Study the drawing (mm; zero at the part's minimum x, y, z) and answer. A direction names the side the tool comes from. Coordinates: 2 decimals unless noted, no trailing zeros. Write each loop counter-clockwise with the first axis right and the second up, starting at its lowest first coordinate (ties: lowest second). Pieces come first, ordered by that corner, then holes. Notation, with made-up numbers: M 77.25,78.5 L 120.25,78.5 A20 cw 120.25,112.5 Z; hole C 79,41 d3. An arc over 180 degrees is marked long. Answer as a JSON object with one key per item and string values. Group by question number.
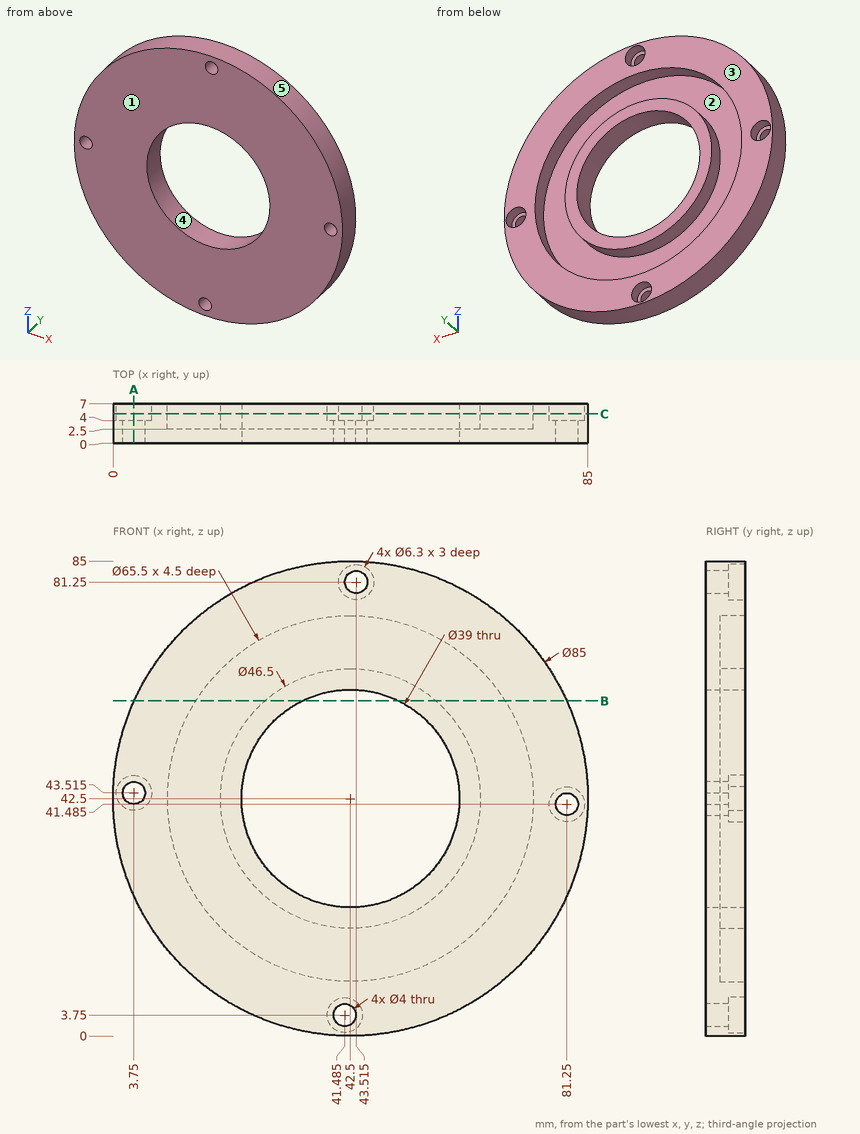
Item 1: A tool of negligible diameter and unlimited length cuts with its end or side. For the marked faces 1 and 2, from which of +Z, -Z, +X, -X, +Y, -Y can it reach the whole face along a straight path? Write none if from no direction.
Item 2: A cutting plane is placed at C-C, the plane y = 5.25. State how many separate pieces and enclosed holes the cut face has, and give its area (3 significant figures).
Item 3: Flat-ended cylindrical pins translate along their axes: pin 1 Ø3 at (x, y) = (29.5, 4.5) entering from +Z (1 decimal); pin 2 Ø1.9 at (x, z) = (42, 81.5) entering from +Y; pin 3 Ø3 at (x, y) = (16, 3) entering from +Z. Find the tip coordinate at first contact, or state that the pin passes through.
Item 4: A cutting plane is placed at B-B, the plane z = 60. Write down the section's boundary in (x, y).
Item 5: For a pull along Z with two mould halves and no side action, classify the marked faces 3, 4 and 5 as +Z half, -Z half, draft (parallel to the pull), parting line (faces both ways), or undercut.
Item 6: A cutting plane is placed at A-A, the plane x = 3.75. Write down the section's boundary in (y, z) (1 decimal).
Item 7: Consider L1, parallel to Z at x = 33.5, y = 3 (1 decimal); L2, parallel to Y at x = 20, z = 30. Determine where each line is inside the solid, lowest interval first. Write a range as from..to.
Answer:
{
 "1": {"face 1": "+Z, -Z, +X, -X, -Y", "face 2": "+Y"},
 "2": {"separate pieces": "2", "enclosed holes": "6", "area": "2,680 mm2"},
 "3": {"pin 1": "z = 83.4", "pin 2": "y = 4", "pin 3": "z = 76.87"},
 "4": {"outline": "M 3.77,0 L 33.9,0 L 33.9,7 L 27.19,7 L 27.19,2.5 L 14.82,2.5 L 14.82,7 L 3.77,7 Z; M 51.1,0 L 81.23,0 L 81.23,7 L 70.18,7 L 70.18,2.5 L 57.81,2.5 L 57.81,7 L 51.1,7 Z"},
 "5": {"face 3": "draft", "face 4": "undercut", "face 5": "parting line"},
 "6": {"outline": "M 0,25 L 7,25 L 7,40.4 L 4,40.4 L 4,41.5 L 0,41.5 Z; M 0,45.5 L 4,45.5 L 4,46.7 L 7,46.7 L 7,60 L 0,60 Z"},
 "7": {"L1": "1..11, 21.1..25.2, 59.8..63.9, 74..84", "L2": "0..2.5"}
}
